Drawing for the job (mm, zero at the part's lowest x, y, z). Coordinates: 2 decimals unless noted, no trailing zeros. Order: outer loops, then holes, each group sorted by start corner. A loop starts at its lowest first (then second) coordinate and runs counter-clockwise, first axis right, second up. Notation, with made-up numbers: (11, -14) - (59, -14) arc R35 cw to (59, 24) - close; hole circle Ø8 at (49, 7). An arc over 180 degrees is marked (long way). Answer as CSV lines item,"result". Start each with the question number.
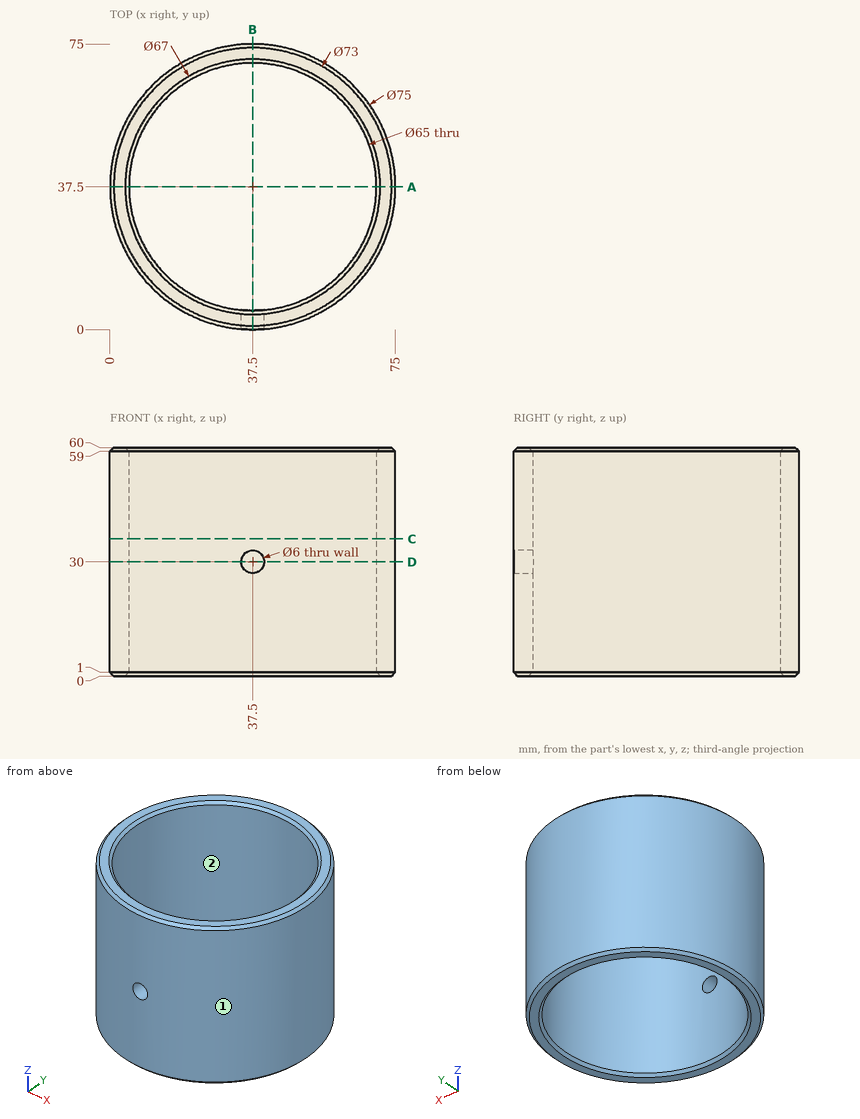
(1) Band-saw the part on B-B on x = 37.5. List the corners of the cut face in (y, z).
(2) Drop flat-ended pins along their axis: pin 1 Ø9.5 at (x, z) = (37.5, 30) entering from +Y; pin 2 Ø2 at (y, z) = (64, 31.5) entering from -X; pin 3 Ø1 at (y, z) = (50, 53) entering from -X; pin 4 Ø5 at (y, z) = (35, 48.5) entering from +X. Give the stop position or say it passes through.
(3) Band-saw the part on A-A on y = 37.5. List the corners of the cut face in (x, z).
(4) Band-saw the part on C-C on z = 36. List the corners of the cut face in (x, y), plus the area to 3 significant figures.
(5) Band-saw the part on D-D on z = 30. List the corners of the cut face in (x, y), plus the area to 3 significant figures.
(6) Probe L1, parallel to Y at x = 37.5, z = 25; L2, parallel to Y at x = 55, z = 9.5. List the from-to ranges inside material, lowest first. Write a range as [from, to].
(7) Pull direction X, two halves, no side cores. Call the marked faces 1 and 2: +X half, -X half, draft (parallel to the pull), parting line (faces both ways), or undercut.
Filled in:
1,outline,"(0, 1) - (1, 0) - (4, 0) - (5, 1) - (5, 27) - (0, 27) - close; (0, 33) - (5, 33) - (5, 59) - (4, 60) - (1, 60) - (0, 59) - close; (70, 1) - (71, 0) - (74, 0) - (75, 1) - (75, 59) - (74, 60) - (71, 60) - (70, 59) - close"
2,pin 1,"stops at y = 75"
2,pin 2,"stops at x = 10"
2,pin 3,"stops at x = 1.97"
2,pin 4,"stops at x = 75"
3,outline,"(0, 1) - (1, 0) - (4, 0) - (5, 1) - (5, 59) - (4, 60) - (1, 60) - (0, 59) - close; (70, 1) - (71, 0) - (74, 0) - (75, 1) - (75, 59) - (74, 60) - (71, 60) - (70, 59) - close"
4,outline,"circle Ø75 at (37.5, 37.5); hole circle Ø65 at (37.5, 37.5)"
4,area,"1,100 mm^2"
5,outline,"(34.5, 0.12) - (34.5, 5.14) arc R32.5 cw (long way) to (40.5, 5.14) - (40.5, 0.12) arc R37.5 ccw (long way) to start"
5,area,"1,070 mm^2"
6,L1,"y = [0, 5], [70, 75]"
6,L2,"y = [4.33, 10.11], [64.89, 70.67]"
7,face 1,"parting line"
7,face 2,"undercut"
